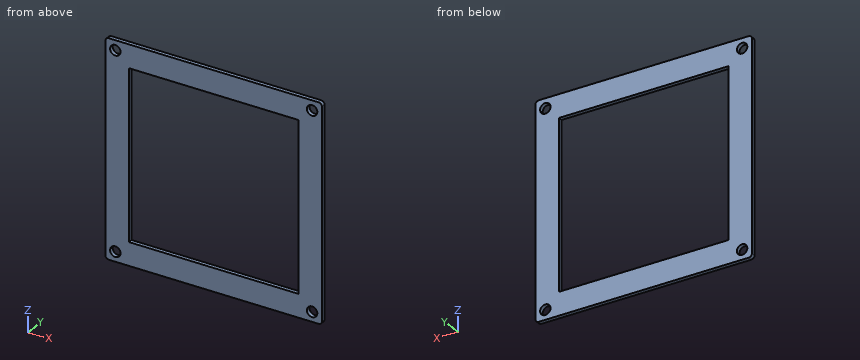
from build123d import *

# Parameters (mm, degrees)
SKETCH1_W           = 66
SKETCH1_H           = 66
SKETCH1_R           = 1.59
SKETCH1_W_2         = 51.8
SKETCH1_H_2         = 51.8
BOSS_EXTRUDE1_DEPTH = 1.27
FILLET1_R           = 1


with BuildPart() as part:
    # Sketch1 → Boss-Extrude1 (new body)
    with BuildSketch(Plane(origin=(0, 0, 0), x_dir=(1, 0, 0), z_dir=(0, 1, 0))):
        Rectangle(SKETCH1_W, SKETCH1_H)
        with Locations(Location((-30, 30, 0), (0, 0, 270))):
            Circle(SKETCH1_R, mode=Mode.SUBTRACT)
        with Locations(Location((30, 30, 0), (0, 0, 270))):
            Circle(SKETCH1_R, mode=Mode.SUBTRACT)
        with Locations(Location((30, -30, 0), (0, 0, 270))):
            Circle(SKETCH1_R, mode=Mode.SUBTRACT)
        with Locations(Location((-30, -30, 0), (0, 0, 270))):
            Circle(SKETCH1_R, mode=Mode.SUBTRACT)
        Rectangle(SKETCH1_W_2, SKETCH1_H_2, mode=Mode.SUBTRACT)
    extrude(amount=BOSS_EXTRUDE1_DEPTH)

    # Fillet1
    fillet1_edges = [part.edges().sort_by_distance(p)[0] for p in [
        (33, 0.635, 33),
        (-33, 0.635, 33),
        (-33, 0.635, -33),
        (33, 0.635, -33),
    ]]
    fillet(fillet1_edges, radius=FILLET1_R)


solid = part.part
For this review, take the finished solid that the model builds, in its own axes (mm). Coordinates: 2 decimals unless noted, no trailing zeros. Order: outer loops, then holes, each group sorted by start corner. A loop starts at its lowest first (then second) coordinate and runs counter-clockwise, first axis right, second up. Notation, with made-up numbers: (49.5, 32.25) - (103.5, 32.25) arc R22 ccw to (103.5, 70.25) - close; hole circle Ø3 at (11, 81). An arc over 180 degrees is marked (long way). Answer as CSV lines item,"result". Start each with the question number.
1) Add section D-D (z = -30). State the section outline as (x, y) points, then the cut area to 3 significant figures.
2) Add section A-A (z = -14). State the section outline as (x, y) points, then the cut area to 3 significant figures.
3) Add section B-B (x = -30). State the section outline as (y, z) points.
4) Add section C-C (y = 0.95). State the section outline as (x, z) points, then the cut area to 3 significant figures.
5) To check wall thickness, follow line 1 along X through (y, z) = (0.6, -30); line 2 along X through (y, z) = (0.65, 5). State the ranges of each line that lie inside material, in increasing order. Write a range as [from, to].
6) Insertion check: P1, Ø10, axis at x = -5, z = 23.5, coming from the +Y side; P2, Ø1.9, axis at x = -30, z = -30, coming from the -Y side. Each pin has a flat end and moves straight along its axis. Give the tip position at first contact, or say it passes through.
Result:
1,outline,"(-33, 0) - (-31.59, 0) - (-31.59, 1.27) - (-33, 1.27) - close; (-28.41, 0) - (28.41, 0) - (28.41, 1.27) - (-28.41, 1.27) - close; (31.59, 0) - (33, 0) - (33, 1.27) - (31.59, 1.27) - close"
1,area,"75.7 mm^2"
2,outline,"(-33, 0) - (-25.9, 0) - (-25.9, 1.27) - (-33, 1.27) - close; (25.9, 0) - (33, 0) - (33, 1.27) - (25.9, 1.27) - close"
2,area,"18.0 mm^2"
3,outline,"(0, -33) - (1.27, -33) - (1.27, -31.59) - (0, -31.59) - close; (0, -28.41) - (1.27, -28.41) - (1.27, 28.41) - (0, 28.41) - close; (0, 31.59) - (1.27, 31.59) - (1.27, 33) - (0, 33) - close"
4,outline,"(-33, -32) arc R1 ccw to (-32, -33) - (32, -33) arc R1 ccw to (33, -32) - (33, 32) arc R1 ccw to (32, 33) - (-32, 33) arc R1 ccw to (-33, 32) - close; hole circle Ø3.18 at (-30, -30); hole circle Ø3.18 at (-30, 30); hole (-25.9, -25.9) - (25.9, -25.9) - (25.9, 25.9) - (-25.9, 25.9) - close; hole circle Ø3.18 at (30, -30); hole circle Ø3.18 at (30, 30)"
4,area,"1,640 mm^2"
5,line 1,"[-33, -31.59], [-28.41, 28.41], [31.59, 33]"
5,line 2,"[-33, -25.9], [25.9, 33]"
6,P1,"y = 1.27"
6,P2,"through"
